from build123d import *

# Parameters (mm, degrees)
SKIZZE1_W                        = 45
SKIZZE1_H                        = 65
AUFSATZ_LINEAR_AUSTRAGEN1_DEPTH  = 38
SKIZZE2_OUTSIDE_W                = 99.932
SKIZZE2_OUTSIDE_H                = 88.932
SCHNITT_LINEAR_AUSTRAGEN1_DEPTH  = 35.4
SCHNITT_LINEAR_AUSTRAGEN2_DEPTH  = 35
SKIZZE4_R                        = 3.3
SCHNITT_LINEAR_AUSTRAGEN3_DEPTH  = 84.030115019
AUFSATZ_LINEAR_AUSTRAGEN2_DEPTH  = 9.6
SKIZZE6_R                        = 16.1
SCHNITT_LINEAR_AUSTRAGEN4_DEPTH  = 7.4
SKIZZE8_R                        = 13
SCHNITT_LINEAR_AUSTRAGEN5_DEPTH  = 185.645606501
SKIZZE9_R                        = 1.5
SCHNITT_LINEAR_AUSTRAGEN6_DEPTH  = 185.645606501
SKIZZE12_W                       = 76
SKIZZE12_H                       = 45
AUFSATZ_LINEAR_AUSTRAGEN4_DEPTH  = 4
SKIZZE10_W                       = 45
SKIZZE10_H                       = 4
AUFSATZ_LINEAR_AUSTRAGEN3_DEPTH  = 18
VERRUNDUNG1_R                    = 15
SKIZZE11_R                       = 2.2
SCHNITT_LINEAR_AUSTRAGEN7_DEPTH  = 183.752564961
VERRUNDUNG1_OF_SPIEGELN1_R       = 15
SKIZZE13_R                       = 3.7
SKIZZE13_R_2                     = 1.7
AUFSATZ_LINEAR_AUSTRAGEN5_DEPTH  = 9.178687268
SCHNITT_LINEAR_START             = -9.6
SKIZZE14_R                       = 1.7
SCHNITT_LINEAR_AUSTRAGEN8_DEPTH  = 9.6
SKIZZE15_R                       = 5
SCHNITT_LINEAR_AUSTRAGEN9_DEPTH  = 9.6
SKIZZE19_R                       = 3.25
SCHNITT_LINEAR_AUSTRAGEN11_DEPTH = 3.4
VERRUNDUNG2_R                    = 10
FASE2_SIZE                       = 2
VERRUNDUNG3_R                    = 2.5


with BuildPart() as part:
    # Skizze1 → Aufsatz-Linear austragen1 (new, symmetric)
    with BuildSketch(Plane(origin=(0, 0, 0), x_dir=(0, 0, -1), z_dir=(1, 0, 0))):
        with Locations((0, 32.5)):
            Rectangle(SKIZZE1_W, SKIZZE1_H)
    extrude(amount=AUFSATZ_LINEAR_AUSTRAGEN1_DEPTH, both=True)

    # Skizze2 outside → Schnitt-Linear austragen1 (cut)
    with BuildSketch(Plane.XY.offset(22.5)):
        with Locations((0, 32.5)):
            Rectangle(SKIZZE2_OUTSIDE_W, SKIZZE2_OUTSIDE_H)
        Polygon((-38, 0), (-28, 0), (-22.226497308, 10), (-28, 20), (-28, 45), (-22.226497308, 55), (-28, 65), (-38, 65), align=None, mode=Mode.SUBTRACT)
        Polygon((38, 65), (38, 0), (28, 0), (22.226497308, 10), (28, 20), (28, 45), (22.226497308, 55), (28, 65), align=None, mode=Mode.SUBTRACT)
    extrude(amount=-SCHNITT_LINEAR_AUSTRAGEN1_DEPTH, mode=Mode.SUBTRACT)

    # Skizze3 → Schnitt-Linear austragen2 (cut)
    with BuildSketch(Plane(origin=(0, 0, -22.5), x_dir=(-1, 0, 0), z_dir=(0, 0, -1))):
        with BuildLine():
            Line((-32, 17.5), (-38, 17.5))
            Line((-38, 17.5), (-38, 2.5))
            Line((-38, 2.5), (-32, 2.5))
            ThreePointArc((-32, 2.5), (-24.5, 10), (-32, 17.5))
        make_face()
        with BuildLine():
            Line((38, 17.5), (38, 2.5))
            Line((38, 2.5), (32, 2.5))
            ThreePointArc((32, 2.5), (24.5, 10), (32, 17.5))
            Line((32, 17.5), (38, 17.5))
        make_face()
        with BuildLine():
            Line((32, 47.5), (38, 47.5))
            Line((38, 47.5), (38, 62.5))
            Line((38, 62.5), (32, 62.5))
            ThreePointArc((32, 62.5), (24.5, 55), (32, 47.5))
        make_face()
        with BuildLine():
            Line((-38, 47.5), (-38, 62.5))
            Line((-38, 62.5), (-32, 62.5))
            ThreePointArc((-32, 62.5), (-24.5, 55), (-32, 47.5))
            Line((-32, 47.5), (-38, 47.5))
        make_face()
    extrude(amount=-SCHNITT_LINEAR_AUSTRAGEN2_DEPTH, mode=Mode.SUBTRACT)

    # Skizze4 → Schnitt-Linear austragen3 (cut, through all)
    with BuildSketch(Plane(origin=(0, 0, 12.5), x_dir=(-1, 0, 0), z_dir=(0, 0, -1))):
        with Locations(Location((32, 10, 0), (0, 0, 90))):
            Circle(SKIZZE4_R)
        with Locations(Location((-32, 10, 0), (0, 0, 270))):
            Circle(SKIZZE4_R)
        with Locations(Location((-32, 55, 0), (0, 0, 90))):
            Circle(SKIZZE4_R)
        with Locations(Location((32, 55, 0), (0, 0, 270))):
            Circle(SKIZZE4_R)
    extrude(amount=-SCHNITT_LINEAR_AUSTRAGEN3_DEPTH, mode=Mode.SUBTRACT)

    # Skizze5 → Aufsatz-Linear austragen2 (add)
    with BuildSketch(Plane.XY.offset(-12.9)):
        with BuildLine():
            Line((-38, 65), (38, 65))
            Line((38, 65), (38, 137))
            ThreePointArc((38, 137), (0, 175), (-38, 137))
            Line((-38, 137), (-38, 65))
        make_face()
    extrude(amount=-AUFSATZ_LINEAR_AUSTRAGEN2_DEPTH)

    # Skizze6 → Schnitt-Linear austragen4 (cut)
    with BuildSketch(Plane.XY.offset(-12.9)):
        with Locations((0, 137)):
            Circle(SKIZZE6_R)
    extrude(amount=-SCHNITT_LINEAR_AUSTRAGEN4_DEPTH, mode=Mode.SUBTRACT)

    # Skizze8 → Schnitt-Linear austragen5 (cut, through all)
    with BuildSketch(Plane(origin=(0, 0, -22.5), x_dir=(-1, 0, 0), z_dir=(0, 0, -1))):
        with Locations(Location((0, 137, 0), (0, 0, 90))):
            Circle(SKIZZE8_R)
    extrude(amount=-SCHNITT_LINEAR_AUSTRAGEN5_DEPTH, mode=Mode.SUBTRACT)

    # Skizze9 → Schnitt-Linear austragen6 (cut, through all)
    with BuildSketch(Plane(origin=(0, 0, -22.5), x_dir=(-1, 0, 0), z_dir=(0, 0, -1))):
        with Locations(Location((12.34288865, 70, 0), (0, 0, 90))):
            Circle(SKIZZE9_R)
        with Locations(Location((14.98779336, 85, 0), (0, 0, 90))):
            Circle(SKIZZE9_R)
        with Locations(Location((17.632698071, 100, 0), (0, 0, 90))):
            Circle(SKIZZE9_R)
        with Locations(Location((-12.34288865, 70, 0), (0, 0, 180))):
            Circle(SKIZZE9_R)
        with Locations(Location((-17.632698071, 100, 0), (0, 0, 180))):
            Circle(SKIZZE9_R)
        with Locations(Location((-14.98779336, 85, 0), (0, 0, 180))):
            Circle(SKIZZE9_R)
    extrude(amount=-SCHNITT_LINEAR_AUSTRAGEN6_DEPTH, mode=Mode.SUBTRACT)

    # Skizze12 → Aufsatz-Linear austragen4 (add)
    with BuildSketch(Plane.XZ):
        Rectangle(SKIZZE12_W, SKIZZE12_H)
    extrude(amount=AUFSATZ_LINEAR_AUSTRAGEN4_DEPTH)

    # Skizze10 → Aufsatz-Linear austragen3 (add)
    with BuildSketch(Plane(origin=(38, 0, 0), x_dir=(0, 0, -1), z_dir=(1, 0, 0))):
        with Locations((0, -2)):
            Rectangle(SKIZZE10_W, SKIZZE10_H)
    aufsatz_linear_austragen3 = extrude(amount=AUFSATZ_LINEAR_AUSTRAGEN3_DEPTH)

    # Verrundung1
    verrundung1_edges = [part.edges().sort_by_distance(p)[0] for p in [
        (56, -2, -22.5),
        (56, -2, 22.5),
    ]]
    fillet(verrundung1_edges, radius=VERRUNDUNG1_R)

    # Skizze11 → Schnitt-Linear austragen7 (cut, through all)
    with BuildSketch(Plane(origin=(0, 2.5, 0), x_dir=(1, 0, 0), z_dir=(0, 1, 0))):
        with Locations(Location((47, 10, 0), (0, 0, 180))):
            Circle(SKIZZE11_R)
        with Locations(Location((47, -10, 0), (0, 0, 90))):
            Circle(SKIZZE11_R)
    schnitt_linear_austragen7 = extrude(amount=-SCHNITT_LINEAR_AUSTRAGEN7_DEPTH, mode=Mode.SUBTRACT)

    # Spiegeln1: Aufsatz-Linear austragen3, Schnitt-Linear austragen7 across plane
    add(aufsatz_linear_austragen3.mirror(Plane(origin=(0, 0, 0), x_dir=(0, 0, 1), z_dir=(1, 0, 0))))
    add(schnitt_linear_austragen7.mirror(Plane(origin=(0, 0, 0), x_dir=(0, 0, 1), z_dir=(1, 0, 0))), mode=Mode.SUBTRACT)

    # Verrundung1 of Spiegeln1
    verrundung1_of_spiegeln1_edges = [part.edges().sort_by_distance(p)[0] for p in [
        (-56, -2, -22.5),
        (-56, -2, 22.5),
    ]]
    fillet(verrundung1_of_spiegeln1_edges, radius=VERRUNDUNG1_OF_SPIEGELN1_R)

    # Skizze13 → Aufsatz-Linear austragen5 (add)
    # profile 1 of 4: a face of its own
    with BuildSketch(Plane.XY.offset(-12.9)):
        with Locations(Location((-15.5, 36.65, 0), (0, 0, 180))):
            Circle(SKIZZE13_R)
        with Locations(Location((-15.5, 36.65, 0), (0, 0, 180))):
            Circle(SKIZZE13_R_2, mode=Mode.SUBTRACT)
    # profile 2 of 4: a face of its own
    with BuildSketch(Plane.XY.offset(-12.9)):
        with Locations(Location((15.5, 36.65, 0), (0, 0, 180))):
            Circle(SKIZZE13_R)
        with Locations(Location((15.5, 36.65, 0), (0, 0, 180))):
            Circle(SKIZZE13_R_2, mode=Mode.SUBTRACT)
    # profile 3 of 4: a face of its own
    with BuildSketch(Plane.XY.offset(-12.9)):
        with Locations(Location((15.5, 5.65, 0), (0, 0, 180))):
            Circle(SKIZZE13_R)
        with Locations(Location((15.5, 5.65, 0), (0, 0, 180))):
            Circle(SKIZZE13_R_2, mode=Mode.SUBTRACT)
    # profile 4 of 4: a face of its own
    with BuildSketch(Plane.XY.offset(-12.9)):
        with Locations(Location((-15.5, 5.65, 0), (0, 0, 180))):
            Circle(SKIZZE13_R)
        with Locations(Location((-15.5, 5.65, 0), (0, 0, 180))):
            Circle(SKIZZE13_R_2, mode=Mode.SUBTRACT)
    extrude(amount=AUFSATZ_LINEAR_AUSTRAGEN5_DEPTH)

    # Skizze14 → Schnitt-Linear austragen8 (cut)
    with BuildSketch(Plane.XY.offset(-12.9).offset(SCHNITT_LINEAR_START)):
        with Locations(Location((-15.5, 5.65, 0), (0, 0, 180))):
            Circle(SKIZZE14_R)
        with Locations(Location((15.5, 5.65, 0), (0, 0, 180))):
            Circle(SKIZZE14_R)
        with Locations(Location((15.5, 36.65, 0), (0, 0, 180))):
            Circle(SKIZZE14_R)
        with Locations(Location((-15.5, 36.65, 0), (0, 0, 180))):
            Circle(SKIZZE14_R)
    extrude(amount=SCHNITT_LINEAR_AUSTRAGEN8_DEPTH, mode=Mode.SUBTRACT)

    # Skizze15 → Schnitt-Linear austragen9 (cut)
    with BuildSketch(Plane(origin=(0, 0, -22.5), x_dir=(-1, 0, 0), z_dir=(0, 0, -1))):
        with Locations(Location((0, 21.15, 0), (0, 0, 90))):
            Circle(SKIZZE15_R)
    extrude(amount=-SCHNITT_LINEAR_AUSTRAGEN9_DEPTH, mode=Mode.SUBTRACT)

    # Skizze19 → Schnitt-Linear austragen11 (cut)
    with BuildSketch(Plane(origin=(0, 0, -22.5), x_dir=(-1, 0, 0), z_dir=(0, 0, -1))):
        with Locations(Location((-15.5, 36.65, 0), (0, 0, 90))):
            Circle(SKIZZE19_R)
        with Locations(Location((15.5, 36.65, 0), (0, 0, 90))):
            Circle(SKIZZE19_R)
        with Locations(Location((15.5, 5.65, 0), (0, 0, 90))):
            Circle(SKIZZE19_R)
        with Locations(Location((-15.5, 5.65, 0), (0, 0, 90))):
            Circle(SKIZZE19_R)
    extrude(amount=-SCHNITT_LINEAR_AUSTRAGEN11_DEPTH, mode=Mode.SUBTRACT)

    # Verrundung2
    verrundung2_edges = [part.edges().sort_by_distance(p)[0] for p in [
        (-22.226497308, 55, 4.8),
        (-22.226497308, 10, 4.8),
        (22.226497308, 55, 4.8),
        (22.226497308, 10, 4.8),
    ]]
    fillet(verrundung2_edges, radius=VERRUNDUNG2_R)

    # Fase2
    fase2_edges = [part.edges().sort_by_distance(p)[0] for p in [
        (-16.1, 137, -12.9),
    ]]
    chamfer(fase2_edges, length=FASE2_SIZE)

    # Verrundung3
    verrundung3_edges = [part.edges().sort_by_distance(p)[0] for p in [
        (-38, 0, 0),
        (38, 0, 0),
    ]]
    fillet(verrundung3_edges, radius=VERRUNDUNG3_R - 0.0001)  # a hair under: the kernel refuses the full size


solid = part.part
CAD build for the part. Positions are in the model's coordinates, mm. A direction names the side the tool comes from. Give positions to 0.01 mm unless a question says otherwise; leave off trailing zeros. Loops run counter-clockwise (first coordinate to the right, second up) from the corner with the lowest first, then second, coordinate; pieces in that order, holes last. Notation, with made-up numbers: M -9.5,84 L 37.5,84 A16 cw 37.5,108 Z; hole C 14,-24 d1. An arc over 180 degrees is marked long. Answer in a Markdown table with one row per item. Add a question column.
Item 1: Band-saw the part on A-A on z = 19.5. Give the number of separate pieces and of enclosed holes in the cut face, then the cut area to 3 significant figures.
Item 2: Drop flat-ended pins along their axis: P1, Ø10, axis at y = 23.5, z = -18, coming from the +X side; P2, Ø4, axis at x = -34, y = 53.5, coming from the -Z side; P3, Ø3, axis at x = -31, z = 8.5, coming from the +Y side. Give the stop position or say it passes through.
Item 3: Tool access for faces 1 (the face through (-35, 17.5, -5)), 2 (the face through (35, 47.5, -5)), 3 (the face through (18.722, 36.227, -20.824)), 4 (the face through (26.54, 17.47, 5.05)): list every direction of +Z, -Z, +X, -X, +Y, -Y with a clear straight run to the whole face (end or side of a thin tool).
Item 4: Band-saw the part on C-C on y = 55. Give the cut face in (x, z).
Item 5: Probe probe 1 along X at (y, z) = (55, 15.5); probe 2 along X at (y, z) = (36.65, -21.7); probe 3 along Y at (x, z) = (-34, 2.5). List the from-to ranges inside material, lowest first.
Item 6: Band-saw the part on B-B on x = 0. Give the cut face in (y, z).
Reply:
| question | item | result |
|---|---|---|
| 1 | separate pieces | 1 |
| 1 | enclosed holes | 4 |
| 1 | area | 1,780 mm^2 |
| 2 | P1 | stops at x = 38 |
| 2 | P2 | stops at z = 12.5 |
| 2 | P3 | stops at y = 65 |
| 3 | face 1 | -Z, -X |
| 3 | face 2 | -Z, +X |
| 3 | face 3 | -Z |
| 3 | face 4 | +Z |
| 4 | outline | M -38,12.5 L -35.3,12.5 L -35.3,22.5 L -38,22.5 Z; M -28.7,12.5 L -24.5,12.5 L -24.5,-22.5 L 24.5,-22.5 L 24.5,12.5 L 28.7,12.5 L 28.7,22.5 L 23.77,22.5 L 23.77,-12.9 L -23.77,-12.9 L -23.77,22.5 L -28.7,22.5 Z; M 35.3,12.5 L 38,12.5 L 38,22.5 L 35.3,22.5 Z |
| 5 | probe 1 | x = -38 to -35.3, -28.7 to -23.77, 23.77 to 28.7, 35.3 to 38 |
| 5 | probe 2 | x = -38 to -18.75, -12.25 to 12.25, 18.75 to 38 |
| 5 | probe 3 | y = -4 to 2.5, 17.5 to 47.5, 62.5 to 65 |
| 6 | outline | M -4,-22.5 L 16.15,-22.5 L 16.15,-12.9 L 0,-12.9 L 0,22.5 L -4,22.5 Z; M 26.15,-22.5 L 124,-22.5 L 124,-20.3 L 120.9,-20.3 L 120.9,-14.9 L 118.9,-12.9 L 26.15,-12.9 Z; M 150,-22.5 L 175,-22.5 L 175,-12.9 L 155.1,-12.9 L 153.1,-14.9 L 153.1,-20.3 L 150,-20.3 Z |
